Input: dimensioned drawing with shaded views. Units: mm. Origin: part minimum x, y, z. A direction names the side the tool comes from. Coordinates: 2 decimals unless noted, no trailing zeros. Order: outer loops, then holes, each group sorted by start corner. A loop starts at its lowest first (then second) coordinate and runs counter-clockwise, first axis right, second up. Notation, with made-up numbers: (27.25, 3.5) - (42.25, 3.5) arc R28 cw to (42.25, 35.5) - close; hole circle Ø7 at (-25.5, 32.25). An arc over 180 degrees is marked (long way). One line per question, with ' | ' between items. Start each with the question number.
(1) Section A-A (x = 8.75). Return the cut outline in (y, z).
(2) Line query: line 1 along Y through (x, z) = (8.75, 7.75); line 2 along Y through (x, z) = (8.75, 4.25); line 3 along X through (y, z) = (6.25, 5.75). Output: solid intervals per line, ascending.
(3) Draft query along Y for the marked faces 1, 2 and 3. Return one class per face: +Y half, -Y half, draft (parallel to the pull), parting line (faces both ways), or undercut.
(4) Contact query for flat-ended pins moving along their axis: P1, Ø2, axis at y = 11.5, z = 8.5, coming from the -X side (3 decimals); P2, Ø1.5, axis at x = 9.5, z = 2.5, coming from the +Y side; P3, Ø2, axis at y = 10.5, z = 4.5, coming from the -X side. Output: stop coordinate, or through.
(5) Section C-C (z = 5). Return the cut outline in (x, y), then the cut area to 3 significant figures.
(6) Section D-D (y = 16.25). Return the cut outline in (x, z).
(7) Access query for the marked faces 4 and 5. Directions: +Z, -Z, +X, -X, +Y, -Y. A direction counts if a zero-diameter tool reaches every point of the face in a straight line with its end or side. Return the directions, or none.
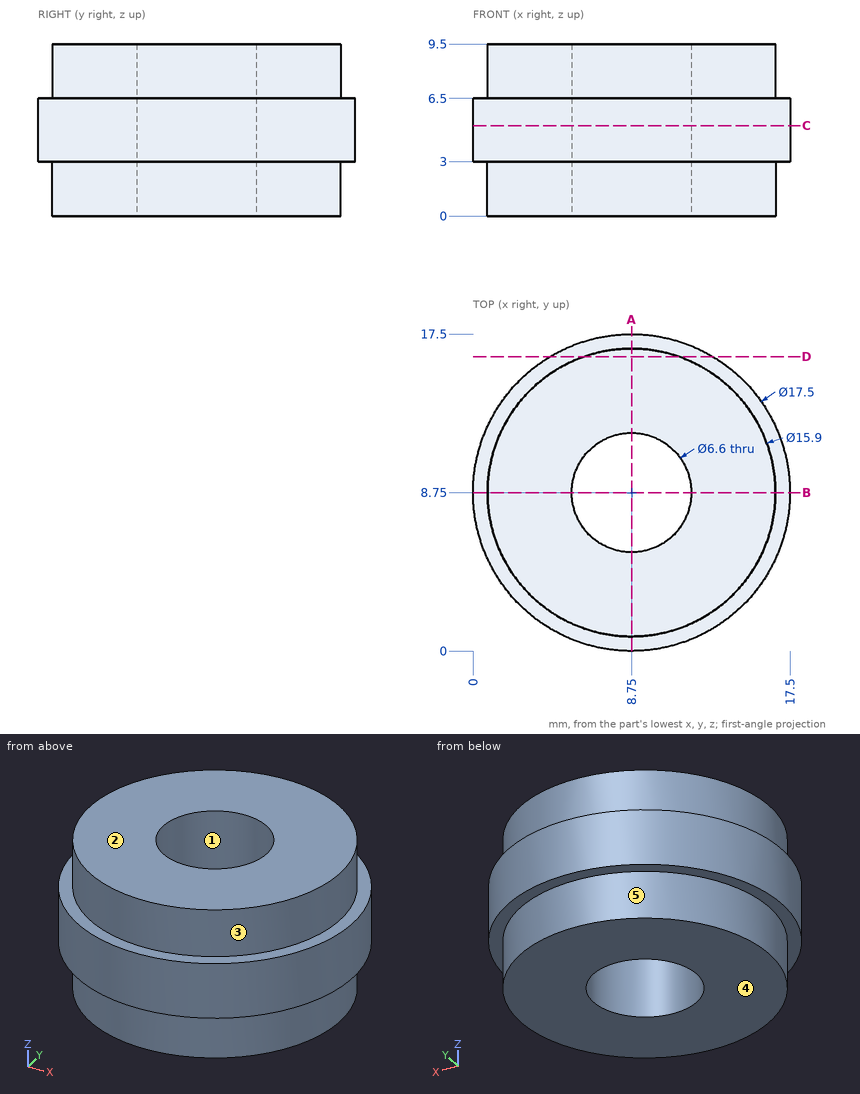
Response values:
1) outline: (0, 3) - (0.8, 3) - (0.8, 0) - (5.45, 0) - (5.45, 9.5) - (0.8, 9.5) - (0.8, 6.5) - (0, 6.5) - close; (12.05, 0) - (16.7, 0) - (16.7, 3) - (17.5, 3) - (17.5, 6.5) - (16.7, 6.5) - (16.7, 9.5) - (12.05, 9.5) - close
2) line 1: y = 0.8 to 5.45, 12.05 to 16.7 | line 2: y = 0 to 5.45, 12.05 to 17.5 | line 3: x = 0.36 to 6.6, 10.9 to 17.14
3) face 1: undercut | face 2: draft | face 3: parting line
4) P1: stops at x = 0.995 | P2: stops at y = 17.5 | P3: stops at x = 0.03
5) outline: circle Ø17.5 at (8.75, 8.75); hole circle Ø6.6 at (8.75, 8.75) | area: 206 mm²
6) outline: (4.24, 3) - (6.11, 3) - (6.11, 0) - (11.39, 0) - (11.39, 3) - (13.26, 3) - (13.26, 6.5) - (11.39, 6.5) - (11.39, 9.5) - (6.11, 9.5) - (6.11, 6.5) - (4.24, 6.5) - close
7) face 4: -Z, +X, -X, +Y, -Y | face 5: -Z
